Can you work these out from the model? Positions are in its coordinate system, mm. Round coordinates to 2 decimals unless told otherwise and drop trailing zeros. Loops run counter-clockwise (first coordinate to the right, second up) from the corner with the lowest first, then second, coordinate; pieces in that order, holes last. Notation, with made-up numbers: (25, 41.25) -> (41, 41.25) arc R12 cw to (41, 51.25) -> close; hole circle Ø7 at (64.5, -28). An arc over 180 degrees is marked (long way). Answer as a JSON object with one key per item and string values.
```python
from build123d import *

# Parameters (mm, degrees)
SKETCH_1_W          = 75
SKETCH_1_H          = 60
EXTRUDE_1_DEPTH     = 1
SKETCH_2_R          = 1.5
CUT_EXTRUDE_1_DEPTH = 49.033842236


with BuildPart() as part:
    # 草图1 → 凸台-拉伸1 (new body)
    with BuildSketch(Plane(origin=(0, 0, 0), x_dir=(1, 0, 0), z_dir=(0, 1, 0))):
        Rectangle(SKETCH_1_W, SKETCH_1_H)
    extrude(amount=EXTRUDE_1_DEPTH)

    # 草图2 → 切除-拉伸1 (cut, through all)
    with BuildSketch(Plane(origin=(0, 0, 0), x_dir=(1, 0, 0), z_dir=(0, 1, 0))):
        with Locations(Location((-32.5, 25, 0), (0, 0, 270))):
            Circle(SKETCH_2_R)
        with Locations(Location((-32.5, -25, 0), (0, 0, 90))):
            Circle(SKETCH_2_R)
        with Locations(Location((32.5, -25, 0), (0, 0, 270))):
            Circle(SKETCH_2_R)
        with Locations(Location((32.5, 25, 0), (0, 0, 90))):
            Circle(SKETCH_2_R)
        with Locations(Location((0, -25, 0), (0, 0, 90))):
            Circle(SKETCH_2_R)
        with Locations(Location((0, 25, 0), (0, 0, 90))):
            Circle(SKETCH_2_R)
    extrude(amount=CUT_EXTRUDE_1_DEPTH, mode=Mode.SUBTRACT)


solid = part.part
```
Q1. I want a section at B-B, the plane z = -25. Write out the boundary of the cut face in (x, y).
Determined:
{"outline": "(-37.5, 0) -> (-34, 0) -> (-34, 1) -> (-37.5, 1) -> close; (-31, 0) -> (-1.5, 0) -> (-1.5, 1) -> (-31, 1) -> close; (1.5, 0) -> (31, 0) -> (31, 1) -> (1.5, 1) -> close; (34, 0) -> (37.5, 0) -> (37.5, 1) -> (34, 1) -> close"}
Q2. We'd pull the mould along Z, two halves only. Please class faces 1 (the cylindrical face through (31.6, 0.5, 23.8)), 2 (the cylindrical face through (33.4, 0.5, -23.8)), 3 (the flat face through (-1, 0, 0)): pulls with the +Z half, pulls with the -Z half, needs draft (parallel to the pull), parting line crosses it, or undercut.
Determined:
{"face 1": "undercut", "face 2": "undercut", "face 3": "needs draft"}
Q3. If I drill on L1, parallel to X at y = 0.35, z = -25; L2, parallel to Z at x = 32.5, y = 0.2; L3, parallel to X at y = 0.25, z = -24, over which ranges is the centre line in solid material (lowest first)? Write a range as [from, to].
Determined:
{"L1": "[-37.5, -34], [-31, -1.5], [1.5, 31], [34, 37.5]", "L2": "[-30, -26.5], [-23.5, 23.5], [26.5, 30]", "L3": "[-37.5, -33.62], [-31.38, -1.12], [1.12, 31.38], [33.62, 37.5]"}
Q4. I want a section at A-A, the plane x = 32.5. Write out the boundary of the cut face in (y, z).
Determined:
{"outline": "(0, -30) -> (1, -30) -> (1, -26.5) -> (0, -26.5) -> close; (0, -23.5) -> (1, -23.5) -> (1, 23.5) -> (0, 23.5) -> close; (0, 26.5) -> (1, 26.5) -> (1, 30) -> (0, 30) -> close"}
